from build123d import *

# Parameters (mm, degrees)
F0_W     = 43
F0_H     = 50
F1_DEPTH = 6
F3_D     = 3.3
F4_DEPTH = 3
F5_D     = 4


with BuildPart() as f1:
    # F0 (on Top) → F1 (new body)
    with BuildSketch(Plane.XY):
        Rectangle(F0_W, F0_H)
    extrude(amount=F1_DEPTH)

    # F3 (through all)
    with Locations(Plane.XY.offset(6)):
        with Locations((-8, 0), (8, 0), (0, 8), (0, -8), (-12, 16), (-12, -16), (12, -16), (12, 16)):
            Hole(F3_D / 2)

    # F2 (on face) → F4 (cut)
    with BuildSketch(Plane.XY.offset(6)):
        Polygon((-20.0207259422, -25), (-15.9792740578, -25), (-13.9585481157, -21.5), (-15.9792740578, -18), (-20.0207259422, -18), (-21.5, -20.5621778265), (-21.5, -22.4378221735), align=None)
        Polygon((-21.5, -25), (-20.0207259422, -25), (-21.5, -22.4378221735), align=None)
        Polygon((13.9585481157, -21.5), (15.9792740578, -25), (20.0207259422, -25), (21.5, -22.4378221735), (21.5, -20.5621778265), (20.0207259422, -18), (15.9792740578, -18), align=None)
        Polygon((21.5, -22.4378221735), (20.0207259422, -25), (21.5, -25), align=None)
        Polygon((20.0207259422, 18), (21.5, 20.5621778265), (21.5, 22.4378221735), (20.0207259422, 25), (15.9792740578, 25), (13.9585481157, 21.5), (15.9792740578, 18), align=None)
        Polygon((20.0207259422, 25), (21.5, 22.4378221735), (21.5, 25), align=None)
        Polygon((-21.5, 22.4378221735), (-21.5, 20.5621778265), (-20.0207259422, 18), (-15.9792740578, 18), (-13.9585481157, 21.5), (-15.9792740578, 25), (-20.0207259422, 25), align=None)
        Polygon((-21.5, 25), (-21.5, 22.4378221735), (-20.0207259422, 25), align=None)
    extrude(amount=-F4_DEPTH, mode=Mode.SUBTRACT)

    # F5 (through all)
    with Locations(Plane.XY.offset(6)):
        with Locations((-18, -21.5), (18, -21.5), (18, 21.5), (-18, 21.5)):
            Hole(F5_D / 2)


solid = f1.part
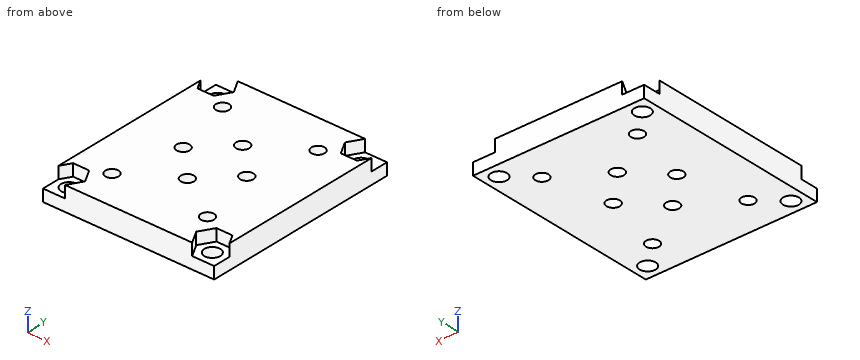
Part model, mm, in its own coordinate system. Give positions to 0.01 mm unless a question says otherwise; leave off trailing zeros. Write each loop counter-clockwise with the first axis right and the second up, starting at its lowest first coordinate (ties: lowest second). Pieces come first, ordered by that corner, then holes.
1) Cut at D-D on x = 0. Write the cut outline in (y, z).
Resolved:
outline: (-25, 0) - (-9.65, 0) - (-9.65, 6) - (-25, 6) - close; (-6.35, 0) - (6.35, 0) - (6.35, 6) - (-6.35, 6) - close; (9.65, 0) - (25, 0) - (25, 6) - (9.65, 6) - close
2) Probe L1, parallel to Y at x = -12, z = 2.2; L2, parallel to Y at x = 18, z = 2.6; L3, parallel to X at y = -14.5, z = 4. List the from-to ranges inside material, lowest first.
Resolved:
L1: y = -25 to -17.65, -14.35 to 14.35, 17.65 to 25
L2: y = -25 to -23.5, -19.5 to 19.5, 23.5 to 25
L3: x = -21.5 to -12.69, -11.31 to 11.31, 12.69 to 21.5
3) Pin check, flat tips, straight feed: pin 1 (6.5 mm diameter, centred on x = 18, y = 21.5, fed in from +Z); pin 2 (2.5 mm diameter, centred on x = 18, y = -21.5, fed in from +Z); pin 3 (0.9 mm diameter, centred on x = -18.5, z = 4, fed in from +Y); pin 4 (1.5 mm diameter, centred on x = -18, z = 4, fed in from -Y). Stop position of each tip, or through.
Resolved:
pin 1: stops at z = 3
pin 2: passes through
pin 3: stops at y = 18
pin 4: stops at y = -18
4) Cut at B-B on z = 3.7. State how many separate pieces and enclosed holes the cut face has, then the cut area to 3 significant figures.
Resolved:
separate pieces: 1
enclosed holes: 8
area: 1,910 mm2
5) Cut at A-A on y = 8. Write the cut outline in (x, z).
Resolved:
outline: (-21.5, 0) - (-1.65, 0) - (-1.65, 6) - (-21.5, 6) - close; (1.65, 0) - (21.5, 0) - (21.5, 6) - (1.65, 6) - close
6) Cut at C-C on y = -16. Write the cut outline in (x, z), then the cut area to 3 significant figures.
Resolved:
outline: (-21.5, 0) - (-13.65, 0) - (-13.65, 6) - (-21.5, 6) - close; (-10.35, 0) - (10.35, 0) - (10.35, 6) - (-10.35, 6) - close; (13.65, 0) - (21.5, 0) - (21.5, 6) - (13.65, 6) - close
area: 218 mm2
